Verification items for the finished model (mm, model axes). A direction names the side the tool comes from. Coordinates: 2 decimals unless noted, no trailing zeros. Loops run counter-clockwise (first coordinate to the right, second up) from the corner with the lowest first, then second, coordinate; pieces in that order, holes last. Notation, with made-up numbers: (57, 71.25) -> (80, 71.25) arc R9 ccw to (80, 83.25) -> close; hole circle Ø9 at (74, 4). An arc over 180 degrees is marked (long way). Write item = value, one per line.
```python
from build123d import *

# Parameters (mm, degrees)
F0_W           = 87.232299149
F0_H           = 65.9088492393
F0_W_2         = 32.4005670846
F0_H_2         = 46.8008210883
F4_D           = 10
F4_CBORE_D     = 15
F4_CBORE_DEPTH = 25


with BuildPart() as f2:
    # F2: sweep along a path in F1
    with BuildLine(Plane.XZ) as f2_path:
        Line((3.3231333364, 0), (19.6618847549, 30.3236078471))
    # F0 (on Top) → F2 (sweep)
    with BuildSketch(Plane.XY):
        Polygon((-40.1545502245, -33.9236706495), (-40.1545502245, 31.9851785898), (47.0777489245, 31.9851785898), (-52.0624481142, 58.2933314145), (-52.0624481142, 11.4925103262), (-84.4630151987, 11.4925103262), align=None)
        with Locations((3.46159935, -0.9692460299)):
            Rectangle(F0_W, F0_H)
        with Locations((-68.2627316564, 34.8929208703)):
            Rectangle(F0_W_2, F0_H_2)
    sweep(path=f2_path.line)

    # F4 (through all)
    with Locations(Plane(origin=(0, 0, 0), x_dir=(1, 0, 0), z_dir=(0, 0, -1))):
        with Locations((-23.7955544144, -10.0916447118)):
            CounterBoreHole(F4_D / 2, F4_CBORE_D / 2, F4_CBORE_DEPTH)


solid = f2.part
```
1) Sectioned sample at A-A, the plane z = 3.5. Record the cut outline in (x, y).
Ans:
outline = (-82.58, 11.49) -> (-38.27, -33.92) -> (48.96, -33.92) -> (48.96, 31.99) -> (-50.18, 58.29) -> (-82.58, 58.29) -> close; hole circle Ø15 at (-23.8, 10.09)
2) Release check for a two-part mould opening along Y. For faces 1 (the face through (55.36, -1.43, 15.37)), 2 (the face through (6.485, 44.955, 15.374)), 3 (the face through (-18.8, 9.9, 27.7)) record: pulls with the +Y half, pulls with the -Y half, needs draft (parallel to the pull), parting line crosses it, or undercut.
Ans:
face_1 = needs draft
face_2 = pulls with the +Y half
face_3 = undercut
3) Sectioned sample at B-B, the plane y = 21. Record the cut outline in (x, z).
Ans:
outline = (-84.46, 0) -> (47.08, 0) -> (63.42, 30.32) -> (-68.12, 30.32) -> close
4) Sectioned sample at C-C, the plane x = -34. Record the cut outline in (y, z).
Ans:
outline = (-33.92, 0) -> (53.5, 0) -> (57.84, 30.32) -> (-23.48, 30.32) -> (-33.92, 11.42) -> close
5) Sectioned sample at D-D, the plane x = 51. Record the cut outline in (y, z), plus the area to 3 significant figures.
Ans:
outline = (-33.92, 7.28) -> (31.99, 7.28) -> (35.28, 30.32) -> (-33.92, 30.32) -> close
area = 1,560 mm2
6) Tool access check on faces 4 (the face through (-19, 12, 25)), 5 (the face through (-60, 58.293, 15)). Record the directions out of +Z, -Z, +X, -X, +Y, -Y that give a thin tool (end or side, any length) a straight path to the whole face; none if there is none.
Ans:
face_4 = -Z
face_5 = +Z, -Z, +X, -X, +Y
7) Depth check by flat-ended pin: pin 1 Ø2 at (x, z) = (-2, 17.5) entering from +Y; pin 2 Ø4 at (y, z) = (-16, 17.5) entering from +X; pin 3 Ø12 at (y, z) = (31.5, 23.5) entering from -X; pin 4 Ø6 at (x, y) = (-23.8, 10.09) entering from -Z. Enter the tip coordinate at first touch or a pass-through.
Ans:
pin_1 = 47.81
pin_2 = 57.58
pin_3 = -75.03
pin_4 = through
8) Material ranges on line 1 (Y direction, x = -28.5, z = 7); line 2 (Y direction, x = -13.5, z = 1); line 3 (X direction, y = 8, z = 29), recorded low to high.
Ans:
line_1 = -33.92 to 4.25, 15.93 to 53.04
line_2 = -33.92 to 48.2
line_3 = -65.43 to -28.34, -19.25 to 62.7
